The listing builds one solid part. Answer for the finished solid, in the listing's coordinates (mm). A direction names the side the tool comes from. Coordinates: 2 decimals unless noted, no trailing zeros. Loops run counter-clockwise (first coordinate to the right, second up) from the corner with the lowest first, then second, coordinate; pieces in that order, holes last. Notation, with made-up numbers: M 66,55 L 87,55 A19 ccw 87,69 Z; hole C -37.75,64.25 d7. An arc over 180 degrees is marked long. Answer in a Markdown table with one row per item. Add a question column.
from build123d import *

# Parameters (mm, degrees)
SKETCH2_R           = 1.6
BOSS_EXTRUDE1_DEPTH = 4.1
CUT_EXTRUDE1_DEPTH  = 2
FILLET4_R           = 30
CUT_EXTRUDE4_DEPTH  = 52.043216983
SKETCH9_W           = 35
SKETCH9_H           = 20
CUT_EXTRUDE5_DEPTH  = 52.043216983


with BuildPart() as part:
    # Sketch2 → Boss-Extrude1 (new body)
    with BuildSketch(Plane(origin=(0, 0, 0), x_dir=(1, 0, 0), z_dir=(0, 1, 0))):
        Polygon((-12.5, 35), (12.5, 35), (23.334523779, 36.062445841), (36.062445841, 23.334523779), (35, 12.5), (35, -12.5), (36.062445841, -23.334523779), (23.334523779, -36.062445841), (12.5, -35), (-12.5, -35), (-23.334523779, -36.062445841), (-36.062445841, -23.334523779), (-35, -12.5), (-35, 12.5), (-36.062445841, 23.334523779), (-23.334523779, 36.062445841), align=None)
        with Locations(Location((22.627416998, 31.112698372, 0), (0, 0, 270))):
            Circle(SKETCH2_R, mode=Mode.SUBTRACT)
        with Locations(Location((31.112698372, 22.627416998, 0), (0, 0, 270))):
            Circle(SKETCH2_R, mode=Mode.SUBTRACT)
        with Locations(Location((22.627416998, -31.112698372, 0), (0, 0, 270))):
            Circle(SKETCH2_R, mode=Mode.SUBTRACT)
        with Locations(Location((31.112698372, -22.627416998, 0), (0, 0, 270))):
            Circle(SKETCH2_R, mode=Mode.SUBTRACT)
        with Locations(Location((-31.112698372, -22.627416998, 0), (0, 0, 270))):
            Circle(SKETCH2_R, mode=Mode.SUBTRACT)
        with Locations(Location((-22.627416998, -31.112698372, 0), (0, 0, 270))):
            Circle(SKETCH2_R, mode=Mode.SUBTRACT)
        with Locations(Location((-22.627416998, 31.112698372, 0), (0, 0, 270))):
            Circle(SKETCH2_R, mode=Mode.SUBTRACT)
        with Locations(Location((-31.112698372, 22.627416998, 0), (0, 0, 270))):
            Circle(SKETCH2_R, mode=Mode.SUBTRACT)
    extrude(amount=BOSS_EXTRUDE1_DEPTH)

    # Sketch4 → Cut-Extrude1 (cut)
    with BuildSketch(Plane(origin=(0, 4.1, 0), x_dir=(1, 0, 0), z_dir=(0, 1, 0))):
        Polygon((29, 12.012193309), (12.012193309, 29), (-12.012193309, 29), (-29, 12.012193309), (-29, -12.012193309), (-12.012193309, -29), (12.012193309, -29), (29, -12.012193309), align=None)
    extrude(amount=-CUT_EXTRUDE1_DEPTH, mode=Mode.SUBTRACT)

    # Fillet4
    # the kernel refuses this fillet: 30 mm, written as the material it adds along each edge
    with BuildSketch(Plane(origin=(35, 0, -12.5), x_dir=(0.09759304388629828, 0, -0.9952264052892723), z_dir=(0, 1, 0)), Plane(origin=(35, 0, 12.5), x_dir=(0, 0, -1), z_dir=(0, 1, 0)), Plane(origin=(12.5, 0, 35), x_dir=(0.9952264052892723, 0, 0.09759304388629875), z_dir=(0, 1, 0)), Plane(origin=(-12.5, 0, 35), x_dir=(1, 0, 0), z_dir=(0, 1, 0)), Plane(origin=(-35, 0, 12.5), x_dir=(-0.09759304388630283, 0, 0.9952264052892719), z_dir=(0, 1, 0)), Plane(origin=(-35, 0, -12.5), x_dir=(0, 0, 1), z_dir=(0, 1, 0)), Plane(origin=(12.5, 0, -35), x_dir=(-1, 0, 0), z_dir=(0, 1, 0))) as fillet4_piece_1:
        with BuildLine():
            CenterArc((FILLET4_R * 0.0489132680019, -FILLET4_R), FILLET4_R, 90, 5.600584003)
            Line((-FILLET4_R * 0.0486797758844, -FILLET4_R * 0.00477359471073), (0, 0))
            Line((0, 0), (FILLET4_R * 0.0489132680019, 0))
        make_face()
    extrude(amount=4.1)
    with BuildSketch(Plane(origin=(-12.5, 0, -35), x_dir=(1, 0, 0), z_dir=(0, 1, 0))) as fillet4_piece_2:
        with BuildLine():
            CenterArc((FILLET4_R * 0.0489132680019, FILLET4_R), FILLET4_R, 264.399415997, 5.600584003)
            Line((-FILLET4_R * 0.0486797758844, FILLET4_R * 0.00477359471073), (0, 0))
            Line((0, 0), (FILLET4_R * 0.0489132680019, 0))
        make_face()
    extrude(amount=4.1)

    # Sketch8 → Cut-Extrude4 (cut, through all)
    with BuildSketch(Plane(origin=(0, 2.1, 0), x_dir=(1, 0, 0), z_dir=(0, 1, 0))):
        with BuildLine():
            Line((-1.5, 19.7), (-1.5, 18.3))
            ThreePointArc((-1.5, 18.3), (-1.734314575, 17.734314575), (-2.3, 17.5))
            Line((-2.3, 17.5), (-6.7, 17.5))
            ThreePointArc((-6.7, 17.5), (-7.265685425, 17.734314575), (-7.5, 18.3))
            Line((-7.5, 18.3), (-7.5, 26.7))
            ThreePointArc((-7.5, 26.7), (-7.265685425, 27.265685425), (-6.7, 27.5))
            Line((-6.7, 27.5), (6.7, 27.5))
            ThreePointArc((6.7, 27.5), (7.265685425, 27.265685425), (7.5, 26.7))
            Line((7.5, 26.7), (7.5, 18.3))
            ThreePointArc((7.5, 18.3), (7.265685425, 17.734314575), (6.7, 17.5))
            Line((6.7, 17.5), (2.3, 17.5))
            ThreePointArc((2.3, 17.5), (1.734314575, 17.734314575), (1.5, 18.3))
            Line((1.5, 18.3), (1.5, 19.7))
            ThreePointArc((1.5, 19.7), (1.734314575, 20.265685425), (2.3, 20.5))
            Line((2.3, 20.5), (4.2, 20.5))
            ThreePointArc((4.2, 20.5), (4.765685425, 20.734314575), (5, 21.3))
            Line((5, 21.3), (5, 23.7))
            ThreePointArc((5, 23.7), (4.765685425, 24.265685425), (4.2, 24.5))
            Line((4.2, 24.5), (-4.2, 24.5))
            ThreePointArc((-4.2, 24.5), (-4.765685425, 24.265685425), (-5, 23.7))
            Line((-5, 23.7), (-5, 21.3))
            ThreePointArc((-5, 21.3), (-4.765685425, 20.734314575), (-4.2, 20.5))
            Line((-4.2, 20.5), (-2.3, 20.5))
            ThreePointArc((-2.3, 20.5), (-1.734314575, 20.265685425), (-1.5, 19.7))
        make_face()
        with BuildLine():
            Line((-7.5, -18.3), (-7.5, -26.7))
            ThreePointArc((-7.5, -26.7), (-7.265685425, -27.265685425), (-6.7, -27.5))
            Line((-6.7, -27.5), (6.7, -27.5))
            ThreePointArc((6.7, -27.5), (7.265685425, -27.265685425), (7.5, -26.7))
            Line((7.5, -26.7), (7.5, -18.3))
            ThreePointArc((7.5, -18.3), (7.265685425, -17.734314575), (6.7, -17.5))
            Line((6.7, -17.5), (2.3, -17.5))
            ThreePointArc((2.3, -17.5), (1.734314575, -17.734314575), (1.5, -18.3))
            Line((1.5, -18.3), (1.5, -19.7))
            ThreePointArc((1.5, -19.7), (1.734314575, -20.265685425), (2.3, -20.5))
            Line((2.3, -20.5), (4.2, -20.5))
            ThreePointArc((4.2, -20.5), (4.765685425, -20.734314575), (5, -21.3))
            Line((5, -21.3), (5, -23.7))
            ThreePointArc((5, -23.7), (4.765685425, -24.265685425), (4.2, -24.5))
            Line((4.2, -24.5), (-4.2, -24.5))
            ThreePointArc((-4.2, -24.5), (-4.765685425, -24.265685425), (-5, -23.7))
            Line((-5, -23.7), (-5, -21.3))
            ThreePointArc((-5, -21.3), (-4.765685425, -20.734314575), (-4.2, -20.5))
            Line((-4.2, -20.5), (-2.3, -20.5))
            ThreePointArc((-2.3, -20.5), (-1.734314575, -20.265685425), (-1.5, -19.7))
            Line((-1.5, -19.7), (-1.5, -18.3))
            ThreePointArc((-1.5, -18.3), (-1.734314575, -17.734314575), (-2.3, -17.5))
            Line((-2.3, -17.5), (-6.7, -17.5))
            ThreePointArc((-6.7, -17.5), (-7.265685425, -17.734314575), (-7.5, -18.3))
        make_face()
    extrude(amount=-CUT_EXTRUDE4_DEPTH, mode=Mode.SUBTRACT)

    # Sketch9 → Cut-Extrude5 (cut, through all)
    with BuildSketch(Plane(origin=(0, 2.1, 0), x_dir=(1, 0, 0), z_dir=(0, 1, 0))):
        Rectangle(SKETCH9_W, SKETCH9_H)
    extrude(amount=-CUT_EXTRUDE5_DEPTH, mode=Mode.SUBTRACT)


solid = part.part
(1) The mould has two halves that part along X. Classify faces 5 (the face through (0, 3, 29)), 6 (the face through (35.037, 2.021, -12.519)), 7 (the face through (-35.035, 2.021, -12.478)): released by +X, released by -X, zero draft, split by the parting line, or undercut.
(2) For faces 1 (the face through (-20.387, 3.114, -20.625)), 2 (the face through (5, 1, 22)), 3 (the face through (0, 2, 35)), 4 (the face through (12.478, 2.021, -35.035)), determine the directions among +Z, -Z, +X, -X, +Y, -Y from which every point of the face is accessible in a straight line to the end or side of a thin tool.
(3) A cutting plane is placed at D-D (y = 1.1). State how many separate pieces and enclosed holes the cut face has, plus the area to 3 significant figures.
(4) Each of these flat-tipped pins is pushed along its axis until it touches: pin 1 (1.7 mm diameter, centred on y = 1.5, z = -23.5, fed in from -X); pin 2 (1.5 mm diameter, centred on x = -25, y = 3.5, fed in from -Z); pin 3 (1 mm diameter, centred on y = 0.5, z = 22, fed in from +X); pin 4 (1.5 mm diameter, centred on y = 0.5, z = 19, fed in from -X). Where does it stop, or does it pass through?
(5) A cutting plane is placed at B-B (z = -15). Give the vertices of the cut face in (x, y).
(6) A cutting plane is placed at C-C (x = 26). Give the vertices of the cut face in (y, z).
(7) Straight lines are drawn through the part: line 1 (Z direction, x = 8.5, y = 1.9); line 2 (X direction, y = 1.55, z = 4); line 3 (X direction, y = 2.4, z = 6). For each, find the intervals that lie inside material, in ascending order.
(8) A cutting plane is placed at A-A (x = 9.5). Give the vertices of the cut face in (y, z), plus the area to 3 significant figures.
Solved:
| question | item | result |
|---|---|---|
| 1 | face 5 | undercut |
| 1 | face 6 | released by +X |
| 1 | face 7 | released by -X |
| 2 | face 1 | +Y |
| 2 | face 2 | +Y, -Y |
| 2 | face 3 | +Z, +Y, -Y |
| 2 | face 4 | -Z, +Y, -Y |
| 3 | separate pieces | 1 |
| 3 | enclosed holes | 11 |
| 3 | area | 3,760 mm² |
| 4 | pin 1 | stops at x = -36.06 |
| 4 | pin 2 | stops at z = -35.15 |
| 4 | pin 3 | stops at x = 35.98 |
| 4 | pin 4 | stops at x = -35.71 |
| 5 | outline | M -35.25,0 L 35.25,0 L 35.25,4.1 L 26.01,4.1 L 26.01,2.1 L -26.01,2.1 L -26.01,4.1 L -35.25,4.1 Z |
| 6 | outline | M 0,-33.4 L 4.1,-33.4 L 4.1,-15.01 L 2.1,-15.01 L 2.1,15.01 L 4.1,15.01 L 4.1,33.4 L 0,33.4 Z |
| 7 | line 1 | z = -35 to -10, 10 to 35 |
| 7 | line 2 | x = -35 to -17.5, 17.5 to 35 |
| 7 | line 3 | x = -35 to -29, 29 to 35 |
| 8 | outline | M 0,-35 L 4.1,-35 L 4.1,-29 L 2.1,-29 L 2.1,-10 L 0,-10 Z; M 0,10 L 2.1,10 L 2.1,29 L 4.1,29 L 4.1,35 L 0,35 Z |
| 8 | area | 129 mm² |
